The listing builds one solid part. Answer for the finished solid, in the listing's coordinates (mm). A direction names the side the tool comes from. Coordinates: 2 decimals unless noted, no trailing zeros. Order: outer loops, then holes, each group sorted by start corner. A loop starts at its lowest first (then second) coordinate and runs counter-clockwise, first axis right, second up. Notation, with made-up numbers: (50.5, 54.5) -> (106.5, 54.5) arc R26 cw to (106.5, 74.5) -> close; hole circle Ø7 at (45.5, 18). An arc over 180 degrees is marked (long way). Answer in a Markdown table with one row per item.
```python
from build123d import *

# Parameters (mm, degrees)
F0_W     = 75
F0_H     = 100
F0_W_2   = 35
F0_H_2   = 60
F1_DEPTH = 40
F2_R     = 25
F3_R     = 45
F5_DEPTH = 10


with BuildPart() as f1:
    # F0 (on Right) → F1 (new body, symmetric)
    with BuildSketch(Plane.YZ):
        with Locations((37.5, 50)):
            Rectangle(F0_W, F0_H)
        with Locations((37.5, 50)):
            Rectangle(F0_W_2, F0_H_2, mode=Mode.SUBTRACT)
    extrude(amount=F1_DEPTH, both=True)

    # F2
    f2_edges = [f1.edges().sort_by_distance(p)[0] for p in [
        (0, 55, 80),
        (0, 55, 20),
    ]]
    fillet(f2_edges, radius=F2_R)

    # F3
    f3_edges = [f1.edges().sort_by_distance(p)[0] for p in [
        (0, 75, 100),
        (0, 75, 0),
    ]]
    fillet(f3_edges, radius=F3_R)

    # F4 (on face) → F5 (join)
    with BuildSketch(Plane.XZ):
        with BuildLine():
            ThreePointArc((-26.743521, 34.39074), (9.504213, 9.227778), (19.879071, 52.116415))
            ThreePointArc((19.879071, 52.116415), (11.445172, 90.989948), (-24.74618, 74.483336))
            Line((-24.74618, 74.483336), (-13.094317, 71.610317))
            ThreePointArc((-13.094317, 71.610317), (12.192518, 74.049378), (-5.425539, 55.746998))
            Line((-5.425539, 55.746998), (-5.425539, 47.93552))
            ThreePointArc((-5.425539, 47.93552), (12.14738, 25.869751), (-14.743108, 34.39074))
            Line((-14.743108, 34.39074), (-26.743521, 34.39074))
        make_face()
    extrude(amount=F5_DEPTH)


solid = f1.part
```
(1) Flat-ended cylindrical pins translate along their axes: pin 1 (12 mm diameter, centred on y = 41, z = 32.5, fed in from -X); pin 2 (8.5 mm diameter, centred on y = -7, z = 53.5, fed in from -X); pin 3 (8 mm diameter, centred on x = -19.5, y = -4.5, fed in from +Z); pin 4 (8 mm diameter, centred on x = 27.5, y = 59, fed in from -Z). Find the tip coordinate at first contact, or state that the pin passes through.
Check values:
| item | result |
|---|---|
| pin 1 | through |
| pin 2 | x = -5.43 |
| pin 3 | z = 88.46 |
| pin 4 | z = 7.58 |
(2) A cutting plane is placed at C-C, the plane x = 0. Determine the outline of the cut face in (y, z), then the cut area to 3 significant figures.
Check values:
| item | result |
|---|---|
| outline | (-10, 7.48) -> (0, 7.48) -> (0, 0) -> (30, 0) arc R45 ccw to (75, 45) -> (75, 55) arc R45 ccw to (30, 100) -> (0, 100) -> (0, 93.7) -> (-10, 93.7) -> (-10, 81.7) -> (0, 81.7) -> (0, 54.61) -> (-10, 54.61) -> (-10, 48.97) -> (0, 48.97) -> (0, 19.48) -> (-10, 19.48) -> close; hole (20, 20) -> (30, 20) arc R25 ccw to (55, 45) -> (55, 55) arc R25 ccw to (30, 80) -> (20, 80) -> close |
| area | 5,100 mm² |
(3) A cutting plane is placed at D-D, the plane z = 92. Determine the outline of the cut face in (x, y).
Check values:
| item | result |
|---|---|
| outline | (-40, 0) -> (-9.16, 0) -> (-9.16, -10) -> (9.16, -10) -> (9.16, 0) -> (40, 0) -> (40, 55.61) -> (-40, 55.61) -> close |
(4) For a pull along Z with two mould halves and no side action, classify faces 6 (the flat face through (1, 75, 50)), 7 (the flat face through (1, 15, 100)), 8 (the cylindrical face through (-0.56, 47.871, 27.518)), 9 (the flat face through (1, 15, 0)) as released by +Z, released by -Z, zero draft, split by the parting line, or undercut.
Check values:
| item | result |
|---|---|
| face 6 | zero draft |
| face 7 | released by +Z |
| face 8 | undercut |
| face 9 | released by -Z |
(5) A cutting plane is placed at B-B, the plane z = 77. Determine the outline of the cut face in (x, y).
Check values:
| item | result |
|---|---|
| outline | (-40, 0) -> (-23.96, 0) -> (-23.96, -10) -> (-10.26, -10) -> (-10.26, 0) -> (10.26, 0) -> (10.26, -10) -> (23.96, -10) -> (23.96, 0) -> (40, 0) -> (40, 20) -> (-40, 20) -> close; (-40, 41.87) -> (40, 41.87) -> (40, 69.26) -> (-40, 69.26) -> close |
(6) Find the intervals of material crossed by line 1 along Z through (x, y) = (0, -5); line 2 along Y through (x, z) = (-11, 48.5); line 3 along Y through (x, z) = (-23, 40), in increasing order. Write a range as from..to.
Check values:
| item | result |
|---|---|
| line 1 | 7.48..19.48, 48.97..54.61, 81.7..93.7 |
| line 2 | 0..20, 55..75 |
| line 3 | 0..20, 54.49..74.72 |
(7) A cutting plane is placed at A-A, the plane x = 33. Determine the outline of the cut face in (y, z), then the cut area to 3 significant figures.
Check values:
| item | result |
|---|---|
| outline | (0, 0) -> (30, 0) arc R45 ccw to (75, 45) -> (75, 55) arc R45 ccw to (30, 100) -> (0, 100) -> close; hole (20, 20) -> (30, 20) arc R25 ccw to (55, 45) -> (55, 55) arc R25 ccw to (30, 80) -> (20, 80) -> close |
| area | 4,800 mm² |
(8) Which of the six approach directions +Z, -Z, +X, -X, +Y, -Y give full straight-line access (tool end or side, diameter ignored) to faces 1 (the flat face through (6, -10, 51)), 2 (the flat face through (-40, 12, 51)), 3 (the flat face through (-5.426, -5, 52)), 4 (the cylindrical face through (12.01, -4.93, 90.7)), 5 (the cylindrical face through (-0.56, 47.482, 72.871))?
Check values:
| item | result |
|---|---|
| face 1 | +Z, -Z, +X, -X, -Y |
| face 2 | +Z, -Z, -X, +Y, -Y |
| face 3 | -X, -Y |
| face 4 | -Y |
| face 5 | +X, -X |
